```python
from build123d import *

# Parameters (mm, degrees)
F1_DEPTH       = 4
F3_D           = 3.3
F3_CSINK_D     = 8.96
F3_CSINK_ANGLE = 90
F4_SIZE        = 2
F5_R           = 2


with BuildPart() as f1:
    # F0 (on Top) → F1 (new body, symmetric)
    with BuildSketch(Plane.XY):
        with BuildLine():
            ThreePointArc((-53.8887429237, 51.9443377852), (-48.8887429237, 56.9443377852), (-43.8887429237, 51.9443377852))
            Line((-43.8887429237, 51.9443377852), (-43.8887429237, 46.9949170947))
            Line((-43.8887429237, 46.9949170947), (-33.8887429237, 46.9949170947))
            Line((-33.8887429237, 46.9949170947), (-33.8887429237, 58.9443377852))
            Line((-33.8887429237, 58.9443377852), (-48.8887429237, 58.9443377852))
            ThreePointArc((-48.8887429237, 58.9443377852), (-53.838490392, 56.8940852535), (-55.8887429237, 51.9443377852))
            Line((-55.8887429237, 51.9443377852), (-53.8887429237, 51.9443377852))
        make_face()
    extrude(amount=F1_DEPTH, both=True)

    # F3 (through all)
    with Locations(Plane(origin=(0, 58.9443377852, 0), x_dir=(-1, 0, 0), z_dir=(0, 1, 0))):
        with Locations((38.8887429237, 0)):
            CounterSinkHole(F3_D / 2, F3_CSINK_D / 2, counter_sink_angle=F3_CSINK_ANGLE)

    # F4
    f4_edges = [f1.edges().sort_by_distance(p)[0] for p in [
        (-33.888743, 52.969627, -4),
        (-33.888743, 52.969627, 4),
    ]]
    chamfer(f4_edges, length=F4_SIZE)

    # F5
    f5_edges = [f1.edges().sort_by_distance(p)[0] for p in [
        (-33.888743, 52.969627, 2),
        (-33.888743, 52.969627, -2),
    ]]
    fillet(f5_edges, radius=F5_R)


solid = f1.part
```
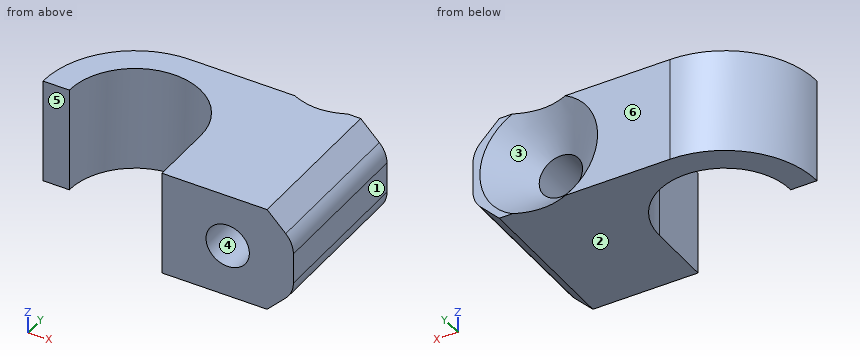
For this review, take the finished solid that the model builds, in its own axes (mm). Face numbers are marked on the shaded views. A direction names the side the tool comes from. Round coordinates to 2 decimals unless told otherwise and drop trailing zeros. Write each loop counter-clockwise with the first axis right and the second up, starting at its lowest first coordinate (ties: lowest second). Pieces come first, ordered by that corner, then holes. Notation, with made-up numbers: M -37,-5.75 L -22,-5.75 A14 cw -22,11.25 Z; hole C 40.25,-3.75 d7. An arc over 180 degrees is marked long. One line per item, written item: value. Start each with the question number.
(1) Wall thickness on line 1 (Z direction, x = -38.75, y = 52.5); line 2 (X direction, y = 52, z = 0); line 3 (X direction, y = 54.25, z = -0.5): over which ranges is each line inside the solid? List them lowest first.
(2) We need section A-A (y = 56.5). Give the boundary of the cut face in (x, z), and give its area (3 significant figures).
(3) Insertion check: pin 1 (2.5 mm diameter, centred on y = 48.5, z = -0.5, fed in from -X); pin 2 (1.6 mm diameter, centred on x = -54.5, z = 1, fed in from -Y); pin 3 (3 mm diameter, centred on x = -51, z = 1, fed in from +Y). Each pin has a flat end and moves straight along its axis. Give the tip position at first contact, or say it passes through.
(4) The part is to be moulded in two halves that separate along Z. For the marked faces 1, 2, 3 and 4, say which applies: released by +Z, released by -Z, zero draft, split by the parting line, or undercut.
(5) Machinability: for the marked faces 5 and 6, which of the approach directions +Z, -Z, +X, -X, +Y, -Y give a long, thin tool a straight path to every point of the face, cutting with its end or side? Answer none if there is none.
(6) We need section C-C (y = 49.75). Give the boundary of the cut face in (x, z).
(7) We need section D-D (y = 55.25). Give the boundary of the cut face in (x, z).
(8) We need section B-B (z = 0). Give the boundary of the cut face in (x, y).
Result:
1. line 1: -4 to -1.64, 1.64 to 4
1. line 2: -55.89 to -53.89, -43.89 to -40.54, -37.24 to -33.89
1. line 3: -55.5 to -53.33, -44.45 to -40.46, -37.32 to -33.89
2. outline: M -54.2,-4 L -50.95,-4 L -50.95,4 L -54.2,4 Z; M -46.83,-4 L -35.89,-4 L -34.47,-2.59 A2 ccw -33.89,-1.17 L -33.89,1.17 A2 ccw -34.47,2.59 L -35.89,4 L -46.83,4 Z; hole C -38.89,0 d4.07
2. area: 112 mm²
3. pin 1: x = -43.89
3. pin 2: y = 51.94
3. pin 3: y = 58.92
4. face 1: zero draft
4. face 2: released by -Z
4. face 3: undercut
4. face 4: undercut
5. face 5: +Z, -Z, -X, -Y
5. face 6: +Z, -Z, +X, -X, +Y
6. outline: M -43.89,-4 L -35.89,-4 L -34.47,-2.59 A2 ccw -33.89,-1.17 L -33.89,1.17 A2 ccw -34.47,2.59 L -35.89,4 L -43.89,4 Z; hole C -38.89,0 d3.3
7. outline: M -55.06,-4 L -52.64,-4 L -52.64,4 L -55.06,4 Z; M -45.14,-4 L -35.89,-4 L -34.47,-2.59 A2 ccw -33.89,-1.17 L -33.89,1.17 A2 ccw -34.47,2.59 L -35.89,4 L -45.14,4 Z; hole C -38.89,0 d3.3
8. outline: M -55.89,51.94 L -53.89,51.94 A5 cw -43.89,51.94 L -43.89,46.99 L -40.54,46.99 L -40.54,56.11 L -43.37,58.94 L -48.89,58.94 A7 ccw Z; M -37.24,46.99 L -33.89,46.99 L -33.89,58.94 L -34.41,58.94 L -37.24,56.11 Z
